```python
from build123d import *

# Parameters (mm, degrees)
CUT_EXTRUDE_1_DEPTH = 10
SKETCH_3_R          = 2
CUT_EXTRUDE_2_DEPTH = 16.5


with BuildPart() as part:
    # Эскиз1 → Повернуть1 (revolve)
    with BuildSketch(Plane.XY):
        Polygon((0, 15.5), (2.5, 15.5), (3, 12), (3, 0), (0, 0), align=None)
    revolve(axis=Axis((0, 0, 0), (0, 1, 0)))

    # Эскиз2 → Вырез-Вытянуть1 (cut)
    with BuildSketch(Plane(origin=(0, 15.5, 0), x_dir=(1, 0, 0), z_dir=(0, 1, 0))):
        Polygon((-0.25, 6.25), (0.25, 6.25), (0.25, 0.25), (6.25, 0.25), (6.25, -0.25), (0.25, -0.25), (0.25, -6.25), (-0.25, -6.25), (-0.25, -0.25), (-6.25, -0.25), (-6.25, 0.25), (-0.25, 0.25), align=None)
    extrude(amount=-CUT_EXTRUDE_1_DEPTH, mode=Mode.SUBTRACT)

    # Эскиз3 → Вырез-Вытянуть2 (cut, through all)
    with BuildSketch(Plane.XZ):
        Circle(SKETCH_3_R)
    extrude(amount=-CUT_EXTRUDE_2_DEPTH, mode=Mode.SUBTRACT)


solid = part.part
```
Build history of the part. All positions in model axes, mm. A direction names the side the tool comes from. Give positions to 0.01 mm unless a question says otherwise; leave off trailing zeros. Loops run counter-clockwise (first coordinate to the right, second up) from the corner with the lowest first, then second, coordinate; pieces in that order, holes last. Notation, with made-up numbers: (6, 55) - (19, 55) arc R16 ccw to (19, 62) - close; hole circle Ø11 at (73, 88.5). An arc over 180 degrees is marked (long way). Use a Markdown table: item, result.
(1) Band-saw the part on B-B (z = 0). Give the cut face in (x, y), and give its area (3 significant figures).
Taken from the geometry:
| item | result |
|---|---|
| outline | (-3, 0) - (-2, 0) - (-2, 5.5) - (-3, 5.5) - close; (2, 0) - (3, 0) - (3, 5.5) - (2, 5.5) - close |
| area | 11.0 mm2 |
(2) Band-saw the part on C-C (y = 7.5). Give the cut face in (x, z).
Taken from the geometry:
| item | result |
|---|---|
| outline | (-2.99, -0.25) arc R3 ccw to (-0.25, -2.99) - (-0.25, -1.98) arc R2 cw to (-1.98, -0.25) - close; (-2.99, 0.25) - (-1.98, 0.25) arc R2 cw to (-0.25, 1.98) - (-0.25, 2.99) arc R3 ccw to start; (0.25, -2.99) arc R3 ccw to (2.99, -0.25) - (1.98, -0.25) arc R2 cw to (0.25, -1.98) - close; (0.25, 1.98) arc R2 cw to (1.98, 0.25) - (2.99, 0.25) arc R3 ccw to (0.25, 2.99) - close |
(3) Pull direction Z, two halves, no side cores. Call faces 4 (the face through (-2.5, 10.6, 0.25)), 5 (the face through (-2, 13.7, 1.9)), 6 (the face through (-0.25, 10.6, 2.5)), 7 (the face through (-2.5, 10.6, -0.25)): +Z half, -Z half, draft (parallel to the pull), parting line (faces both ways), or undercut.
Taken from the geometry:
| item | result |
|---|---|
| face 4 | undercut |
| face 5 | +Z half |
| face 6 | draft |
| face 7 | undercut |
(4) Band-saw the part on D-D (y = 2). Give the cut face in (x, z).
Taken from the geometry:
| item | result |
|---|---|
| outline | circle Ø6 at (0, 0); hole circle Ø4 at (0, 0) |
(5) Drop flat-ended pins along their axis: pin 1 Ø0.8 at (x, y) = (-2.5, 9.5) entering from +Z; pin 2 Ø1.1 at (y, z) = (9, 2.5) entering from +X; pin 3 Ø0.5 at (x, y) = (2.5, 11) entering from +Z; pin 4 Ø2.5 at (x, z) = (0, 0) entering from -Y. Give the stop position or say it passes through.
Taken from the geometry:
| item | result |
|---|---|
| pin 1 | z = 2.14 |
| pin 2 | x = 2.28 |
| pin 3 | z = 1.98 |
| pin 4 | through |
(6) Wall check: line 1 along X through (y, z) = (3, 0); line 2 along X through (y, z) = (5, 2.25); line 3 along Z through (x, y) = (-2.1, 8.75). Give the ranges that are in metal, low to high.
Taken from the geometry:
| item | result |
|---|---|
| line 1 | -3 to -2, 2 to 3 |
| line 2 | -1.98 to 1.98 |
| line 3 | -2.14 to -0.25, 0.25 to 2.14 |
(7) Band-saw the part on A-A (x = 0). Give the cut face in (y, z), and give its area (3 significant figures).
Taken from the geometry:
| item | result |
|---|---|
| outline | (0, -3) - (5.5, -3) - (5.5, -2) - (0, -2) - close; (0, 2) - (5.5, 2) - (5.5, 3) - (0, 3) - close |
| area | 11.0 mm2 |
(8) Which spindle directions (+Z, -Z, +X, -X, +Y, -Y) get a long thin tool onto all of the face, cutting with end or side? Do faces 1 (the face through (0.25, 10.6, -2.5)), 2 (the face through (2.5, 10.6, -0.25)), 3 (the face through (1, 0, 2)). Say none if no direction does.
Taken from the geometry:
| item | result |
|---|---|
| face 1 | +Z, -Z, +Y |
| face 2 | +X, -X, +Y |
| face 3 | +Z, -Z, +X, -X, -Y |
